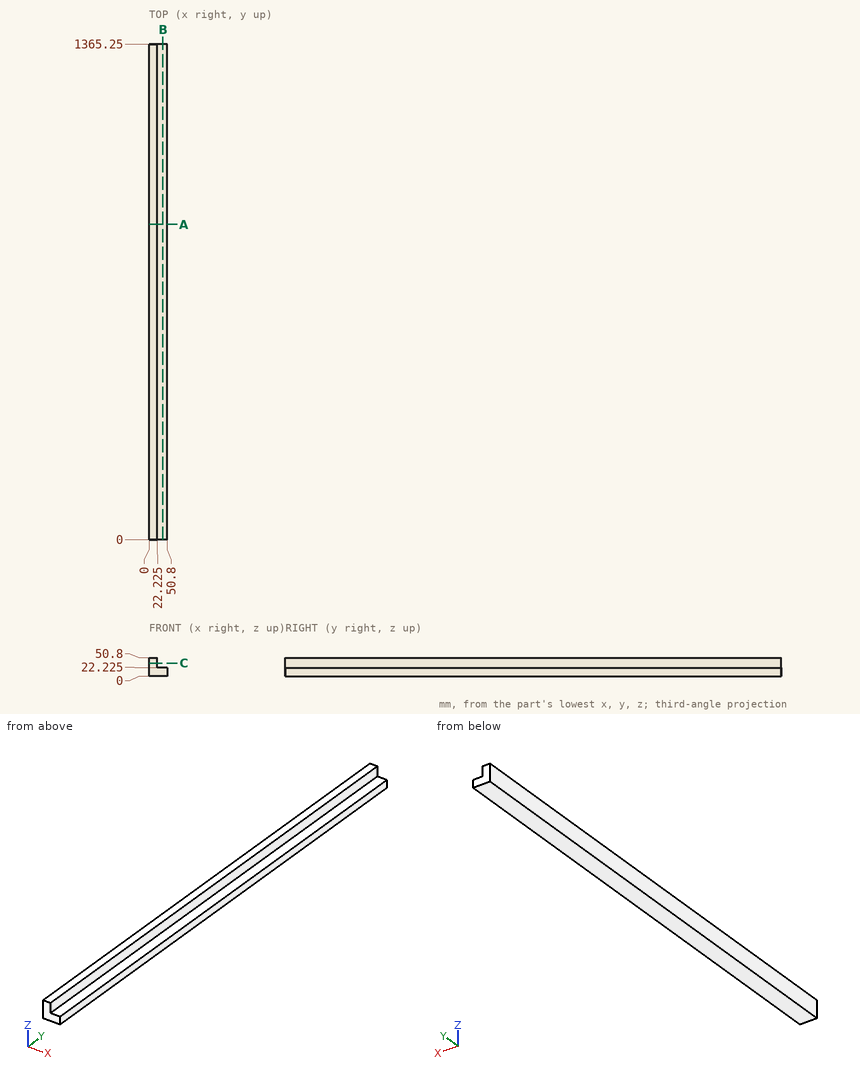
Part print with two shaded views. Sizes in mm from the minimum x, y, z corner. Coordinates: 2 decimals unless noted, no trailing zeros. Order: outer loops, then holes, each group sorted by start corner. A loop starts at its lowest first (then second) coordinate and runs counter-clockwise, first axis right, second up. Notation, with made-up numbers: (0, 9) - (14, 9) arc R25 cw to (14, 45) - close; hole circle Ø6 at (64.5, 80.5). An arc over 180 degrees is marked (long way). Write item = value, one per line. Start each with the question number.
1) Wall check: line 1 along X through (y, z) = (620.5, 39) (3 decimals). Give the ranges that are in metal, low to high. Write a range as from..to.
2) Saw through at A-A on y = 868. Write the cut outline in (x, z) (3 decimals), then the cut area to 3 significant figures.
3) Flat gauge pin, fed straight in: pin 1 Ø12 at (x, y) = (37, 968) entering from +Z (3 decimals). Where does the tip first touch, or does it go through?
4) Saw through at C-C on z = 35.5. Write the cut outline in (x, y) (3 decimals), then the cut area to 3 significant figures.
5) Saw through at B-B on x = 38. Write the cut outline in (y, z) (3 decimals), then the cut area to 3 significant figures.
From the geometry:
q1.line_1 = 0..22.225
q2.outline = (0, 0) - (50.8, 0) - (50.8, 22.225) - (22.225, 22.225) - (22.225, 50.8) - (0, 50.8) - close
q2.area = 1,760 mm^2
q3.pin_1 = 22.225
q4.outline = (0, 0) - (22.225, 0) - (22.225, 1365.25) - (0, 1365.25) - close
q4.area = 30,300 mm^2
q5.outline = (0, 0) - (1365.25, 0) - (1365.25, 22.225) - (0, 22.225) - close
q5.area = 30,300 mm^2
